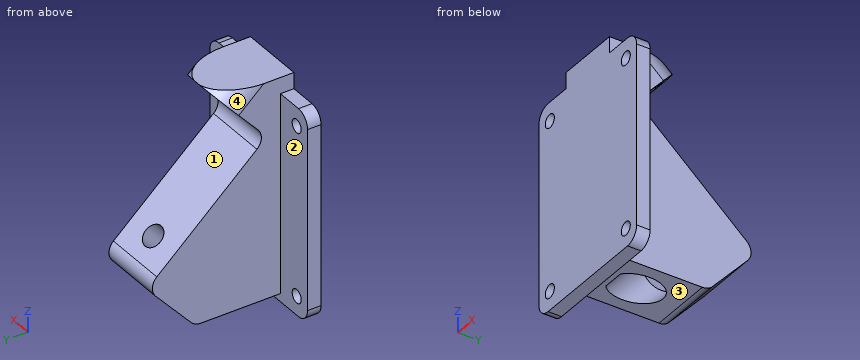
```python
from build123d import *

# Parameters (mm, degrees)
SKETCH1_W                       = 54
SKETCH1_H                       = 77
BOSS_EXTRUDE1_DEPTH             = 5
SKETCH3_W                       = 24
SKETCH3_H                       = 80
BOSS_EXTRUDE2_DEPTH             = 60
BOSS_EXTRUDE2_DIRECTION_2_REACH = 49.289
CUT_EXTRUDE5_DEPTH              = 88.89908987
SKETCH9_R                       = 4
CUT_EXTRUDE7_DEPTH              = 74.599714303
FILLET4_R                       = 5
SKETCH10_R                      = 7.5
CUT_EXTRUDE8_DEPTH              = 20
F_5_0_5_DIAMETER_HOLE1_D        = 5
FILLET7_R                       = 5
CUT_EXTRUDE9_DEPTH              = 79.817150767


with BuildPart() as part:
    # Sketch1 → Boss-Extrude1 (new body)
    with BuildSketch(Plane(origin=(0, 0, 0), x_dir=(1, 0, 0), z_dir=(0, 1, 0))):
        Rectangle(SKETCH1_W, SKETCH1_H)
    extrude(amount=BOSS_EXTRUDE1_DEPTH)

    # Sketch3 → Boss-Extrude2 (add)
    with BuildSketch(Plane(origin=(0, 5, 0), x_dir=(1, 0, 0), z_dir=(0, 1, 0))):
        with Locations((0, -4.5)):
            Rectangle(SKETCH3_W, SKETCH3_H)
    extrude(amount=BOSS_EXTRUDE2_DEPTH)

    # Boss-Extrude2 direction 2: up to this face of the body (flat: up to its plane)
    boss_extrude2_direction_2_end = Plane(part.part.faces().sort_by_distance((0, 0, 0))[0])
    # Sketch3 → Boss-Extrude2 direction 2 (add, up to the picked face)
    with BuildSketch(Plane(origin=(0, 5, 0), x_dir=(1, 0, 0), z_dir=(0, 1, 0)), mode=Mode.PRIVATE) as boss_extrude2_direction_2_sk1:
        with Locations((0, -4.5)):
            Rectangle(SKETCH3_W, SKETCH3_H)
    boss_extrude2_direction_2_tool1 = split(extrude(boss_extrude2_direction_2_sk1.sketch, amount=-BOSS_EXTRUDE2_DIRECTION_2_REACH, mode=Mode.PRIVATE), bisect_by=boss_extrude2_direction_2_end, keep=Keep.BOTH, mode=Mode.PRIVATE)
    add(boss_extrude2_direction_2_tool1.solids().sort_by(Axis((0, 5, 4.5), (0, -1, 0)))[0])

    # Sketch7 → Cut-Extrude5 (cut, through all)
    with BuildSketch(Plane(origin=(12, 0, 0), x_dir=(0, 0, -1), z_dir=(1, 0, 0))):
        Polygon((-46.794344764, 30.073918191), (-24.5, 10), (15.647836382, 54.588689529), (50.5, 23.207660454), (50.5, 70), (-49.5, 70), (-49.5, 27.068983625), align=None)
    extrude(amount=-CUT_EXTRUDE5_DEPTH, mode=Mode.SUBTRACT)

    # Sketch9 → Cut-Extrude7 (cut, through all)
    with BuildSketch(Plane(origin=(0, 16.660250902, 18.503083152), x_dir=(1, 0, 0), z_dir=(0, 0.6691306063588566, 0.7431448254773958))):
        with Locations(Location((0, 37.037748399, 0), (0, 0, 270))):
            Circle(SKETCH9_R)
    extrude(amount=-CUT_EXTRUDE7_DEPTH, mode=Mode.SUBTRACT)

    # Fillet4
    fillet4_edges = [part.edges().sort_by_distance(p)[0] for p in [
        (0, 36.713721119, -35.5),
        (0, 54.588689529, -15.647836382),
        (0, 10, 24.5),
    ]]
    fillet(fillet4_edges, radius=FILLET4_R)

    # Sketch10 → Cut-Extrude8 (cut)
    with BuildSketch(Plane(origin=(0, -13.450626384, -14.938433995), x_dir=(1, 0, 0), z_dir=(0, 0.6691306063588566, 0.7431448254773958))):
        with Locations(Location((0, 37.037748399, 0), (0, 0, 237.266633069))):
            Circle(SKETCH10_R)
    extrude(amount=CUT_EXTRUDE8_DEPTH, mode=Mode.SUBTRACT)

    # Ø5.0 (5) Diameter Hole1 (through all)
    with Locations(Plane(origin=(21, 0, -31.5), x_dir=(0, 0, -1), z_dir=(0, -1, 0))):
        with Locations((0, 0), (0, -42), (-63, -42), (-63, 0)):
            Hole(F_5_0_5_DIAMETER_HOLE1_D / 2)

    # Fillet7
    fillet7_edges = [part.edges().sort_by_distance(p)[0] for p in [
        (27, 2.5, 38.5),
        (-27, 2.5, 38.5),
        (-27, 2.5, -38.5),
        (27, 2.5, -38.5),
    ]]
    fillet(fillet7_edges, radius=FILLET7_R)

    # Sketch8 → Cut-Revolve4 (revolve, cut)
    with BuildSketch(Plane(origin=(0, -6.660250902, 5.996916848), x_dir=(1, 0, 0), z_dir=(0, 0.7431448254773959, -0.6691306063588564))):
        with BuildLine():
            Line((0, -47.898354288), (0, -31.898354288))
            ThreePointArc((0, -31.898354288), (8, -39.898354288), (0, -47.898354288))
        make_face()
    revolve(axis=Axis((0, 28.008080886, 44.5), (0, -0.6691306063588564, -0.7431448254773959)), mode=Mode.SUBTRACT)

    # Sketch13 → Cut-Extrude9 (cut, through all)
    with BuildSketch(Plane(origin=(0, -6.660250902, 5.996916848), x_dir=(1, 0, 0), z_dir=(0, 0.7431448254773957, -0.6691306063588566))):
        with BuildLine():
            Line((-12.01867578, -39.898354288), (-15.599845955, -39.898354288))
            Line((-15.599845955, -39.898354288), (-15.599845955, -55.363727993))
            Line((-15.599845955, -55.363727993), (15.599845955, -55.363727993))
            Line((15.599845955, -55.363727993), (15.599845955, -39.898354288))
            Line((15.599845955, -39.898354288), (11.98132422, -39.898354288))
            ThreePointArc((11.98132422, -39.898354288), (-0.01867578, -51.898354288), (-12.01867578, -39.898354288))
        make_face()
    extrude(amount=-CUT_EXTRUDE9_DEPTH, mode=Mode.SUBTRACT)


solid = part.part
```
Verification items for the finished model (mm, model axes). Face numbers are marked on the shaded views. Coordinates: 2 decimals unless noted, no trailing zeros. Loops run counter-clockwise (first coordinate to the right, second up) from the corner with the lowest first, then second, coordinate; pieces in that order, holes last. Notation, with made-up numbers: (61, 11.25) -> (102, 11.25) arc R4 ccw to (102, 15.25) -> close; hole circle Ø8 at (17.5, 67.5). An arc over 180 degrees is marked (long way). Answer in a Markdown table with one row per item.
1) Draft check along Z on the marked faces 1, 2, 3 and 4. Enter one of: released by +Z, released by -Z, zero draft, split by the parting line, or undercut.
The answers:
| item | result |
|---|---|
| face 1 | undercut |
| face 2 | zero draft |
| face 3 | released by -Z |
| face 4 | released by +Z |
2) Section check A-A (x = -21). Record the cut outline in (y, z), and give its area (3 significant figures).
The answers:
| item | result |
|---|---|
| outline | (0, -38.5) -> (5, -38.5) -> (5, -34) -> (0, -34) -> close; (0, -29) -> (5, -29) -> (5, 29) -> (0, 29) -> close; (0, 34) -> (5, 34) -> (5, 38.5) -> (0, 38.5) -> close |
| area | 335 mm2 |
3) Section check C-C (z = -31.5). Give the number of separate pieces and of enclosed holes in the cut face, and give its area (3 significant figures).
The answers:
| item | result |
|---|---|
| separate pieces | 3 |
| enclosed holes | 1 |
| area | 830 mm2 |
4) Section check B-B (z = 31.5). Record the cut outline in (x, y).
The answers:
| item | result |
|---|---|
| outline | (-27, 0) -> (-23.5, 0) -> (-23.5, 5) -> (-27, 5) -> close; (-18.5, 0) -> (18.5, 0) -> (18.5, 5) -> (12, 5) -> (12, 16.3) -> (5.73, 16.3) arc R6.84 cw to (-5.73, 16.3) -> (-12, 16.3) -> (-12, 5) -> (-18.5, 5) -> close; (23.5, 0) -> (27, 0) -> (27, 5) -> (23.5, 5) -> close |
5) Scan lines: line 1 along X through (y, z) = (3.35, -31.5); line 2 along X through (y, z) = (1, 31); line 3 along Z through (x, y) = (-10, 9.5). Record each from-to range of solid material in increasing order. Write a range as from..to.
The answers:
| item | result |
|---|---|
| line 1 | x = -27..-23.5, -18.5..18.5, 23.5..27 |
| line 2 | x = -27..-23.45, -18.55..18.55, 23.45..27 |
| line 3 | z = -35.5..44.5 |
6) Depth check by flat-ended pin: P1, Ø12, axis at y = 21.5, z = 31, coming from the -X side; P2, Ø5, axis at x = 8, z = -19.5, coming from the +Y side; P3, Ø4, axis at x = 3.5, z = -24, coming from the +Y side. Enter the tip coordinate at first touch or a pass-through.
The answers:
| item | result |
|---|---|
| P1 | stops at x = -12 |
| P2 | stops at y = 52.43 |
| P3 | stops at y = 48.87 |
